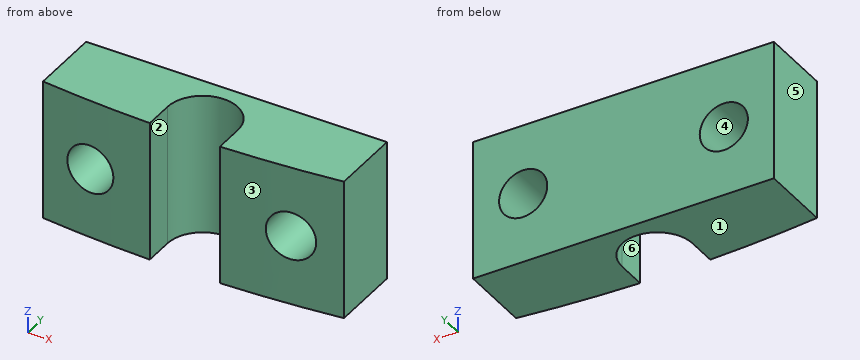
```python
from build123d import *

# Parameters (mm, degrees)
BOSS_EXTRUDE1_DEPTH = 7
SKETCH2_R           = 1.2
CUT_EXTRUDE1_DEPTH  = 10


with BuildPart() as part:
    # Sketch1 → Boss-Extrude1 (new body)
    with BuildSketch(Plane.XY):
        with BuildLine():
            Line((0, 0), (15, 0))
            Line((15, 0), (15, -3.565857851))
            ThreePointArc((15, -3.565857851), (12.037715119, -3.841415326), (9.065924059, -3.981134815))
            Line((9.065924059, -3.981134815), (9.065924059, -2.5))
            ThreePointArc((9.065924059, -2.5), (7.315924059, -0.75), (5.565924059, -2.5))
            Line((5.565924059, -2.5), (5.565924059, -3.971219399))
            ThreePointArc((5.565924059, -3.971219399), (2.778609663, -3.828299941), (0, -3.565857851))
            Line((0, -3.565857851), (0, 0))
        make_face()
    extrude(amount=BOSS_EXTRUDE1_DEPTH)

    # Sketch2 → Cut-Extrude1 (cut)
    with BuildSketch(Plane(origin=(0, 0, 0), x_dir=(1, 0, 0), z_dir=(0, 1, 0))):
        with Locations((12.5, -3.5)):
            Circle(SKETCH2_R)
        with Locations((2.5, -3.5)):
            Circle(SKETCH2_R)
    extrude(amount=-CUT_EXTRUDE1_DEPTH, mode=Mode.SUBTRACT)


solid = part.part
```
Here's how the part is built. I have some questions about the finished solid (model axes, mm). Face numbers are marked on the shaded views. A direction names the side the tool comes from. Give positions to 0.01 mm unless a question says otherwise; leave off trailing zeros. Order: outer loops, then holes, each group sorted by start corner. A loop starts at its lowest first (then second) coordinate and runs counter-clockwise, first axis right, second up. Notation, with made-up numbers: M 32,68.25 L 65,68.25 A15 ccw 65,80.25 Z; hole C -16.75,-30.5 d6. An arc over 180 degrees is marked long. Use a Markdown table: item, result. Add a question column.
1. Suppose I cut it at D-D (y = -0.9). List the corners of the cut face in (x, z) for me.
2. On a 3-axis mill with a long thin cutter (end or side, diameter ignored), from which of +Z, -Z, +X, -X, +Y, -Y can I reach the whole of each face in a straight line? I mean the marked faces 5 and 6. Say none if no direction works.
3. If we mould it in two halves opening along X, with no side actions, what happens to the marked faces 1, 2, 3 and 4? For each: +X half, -X half, draft (parallel to the pull), parting line (faces both ways), or undercut.
4. Suppose I cut it at B-B (x = 2.75). List the corners of the cut face in (y, z) for me.
5. Suppose I cut it at C-C (z = 2.5). List the corners of the cut face in (x, y) for me, and give its area (3 significant figures).
6. I need wall thicknesses on probe 1 along X at (y, z) = (-2.5, 3.5); probe 2 along X at (y, z) = (-3.25, 6.75); probe 3 along Z at (x, y) = (2.5, -2.8). Which ranges of each line are inside material? Lowest first, please. Write a range as from..to.
7. For pin 1 Ø4 at (x, z) = (3.5, 5.5) entering from -Y; pin 2 Ø3 at (x, z) = (12.5, 1.5) entering from -Y, each with a flat end and sliding along its axis, tell me the tip position at first contact or that it passes through.
8. Suppose I cut it at A-A (y = -2.8). List the corners of the cut face in (x, z) for me.
Results list:
| question | item | result |
|---|---|---|
| 1 | outline | M 0,0 L 6.61,0 L 6.61,7 L 0,7 Z; M 8.02,0 L 15,0 L 15,7 L 8.02,7 Z; hole C 2.5,3.5 d2.4; hole C 12.5,3.5 d2.4 |
| 2 | face 5 | +Z, -Z, -X, +Y, -Y |
| 2 | face 6 | +Z, -Z, -Y |
| 3 | face 1 | draft |
| 3 | face 2 | undercut |
| 3 | face 3 | +X half |
| 3 | face 4 | undercut |
| 4 | outline | M -3.83,0 L 0,0 L 0,2.33 L -3.83,2.33 Z; M -3.83,4.67 L 0,4.67 L 0,7 L -3.83,7 Z |
| 5 | outline | M 0,-3.57 A65 ccw 1.84,-3.75 L 1.84,0 L 0,0 Z; M 3.16,-3.86 A65 ccw 5.57,-3.97 L 5.57,-2.5 A1.75 cw 9.07,-2.5 L 9.07,-3.98 A65 ccw 11.84,-3.86 L 11.84,0 L 3.16,0 Z; M 13.16,-3.75 A65 ccw 15,-3.57 L 15,0 L 13.16,0 Z |
| 5 | area | 37.7 mm² |
| 6 | probe 1 | x = 0..1.3, 3.7..5.57, 9.07..11.3, 13.7..15 |
| 6 | probe 2 | x = 0..5.57, 9.07..15 |
| 6 | probe 3 | z = 0..2.3, 4.7..7 |
| 7 | pin 1 | stops at y = -3.97 |
| 7 | pin 2 | stops at y = -3.91 |
| 8 | outline | M 0,0 L 5.57,0 L 5.57,7 L 0,7 Z; M 9.07,0 L 15,0 L 15,7 L 9.07,7 Z; hole C 2.5,3.5 d2.4; hole C 12.5,3.5 d2.4 |
